Can you work these out from the model? Positions are in its coordinate system, mm. Round coordinates to 2 decimals unless told otherwise and drop trailing zeros. One line per question, with ' | ' between items.
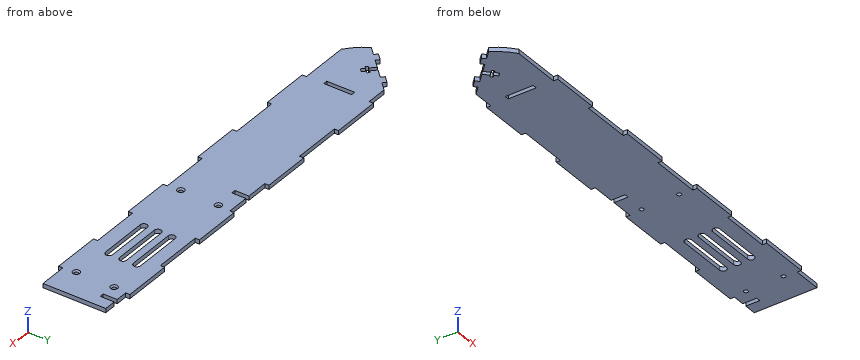
Autodesk Inventor part; units mm, degrees
ref_plane "YZ Plane" through (0, 0, 0) normal (1, 0, 0) x (0, 1, 0)
ref_plane "XZ Plane" through (0, 0, 0) normal (0, 1, 0) x (-1, 0, 0)
ref_plane "XY Plane" through (0, 0, 0) normal (0, 0, 1) x (1, 0, 0)
sketch "Sketch1" plane through (0, 0, 0) normal (0, 0, 1) x (1, 0, 0)
  line L0 (142.5, -22.5) -> (142.5, 22.5)
  arc A0 (-169.3198, -9.3198) -> (-157.5, -22.5) centre (-130.5627, 13.547) ccw
  line L1 (-154.4706, 5.5294) -> (-150.935, 1.9939)
  line L2 (-150.935, 1.9939) -> (-152.2157, 0.7132)
  line L3 (-152.2157, 0.7132) -> (-150.8015, -0.701)
  line L4 (-150.8015, -0.701) -> (-149.5208, 0.5797)
  line L5 (-149.5208, 0.5797) -> (-147.3995, -1.5416)
  line L6 (-147.3995, -1.5416) -> (-145.2782, 0.5797)
  line L7 (-145.2782, 0.5797) -> (-147.3995, 2.701)
  line L8 (-147.3995, 2.701) -> (-146.1188, 3.9817)
  line L9 (-146.1188, 3.9817) -> (-147.533, 5.3959)
  line L10 (-147.533, 5.3959) -> (-148.8137, 4.1152)
  line L11 (-148.8137, 4.1152) -> (-152.3492, 7.6508)
  line L12 (-154.542, 7.7222) -> (-156.666, 9.8462) construction
  line L13 (-122.5, 22.5) -> (-122.5, 25.5)
  line L14 (-122.5, 25.5) -> (-87.5, 25.5)
  line L15 (-87.5, 25.5) -> (-87.5, 22.5)
  line L16 (-52.5, 22.5) -> (-52.5, 25.5)
  line L17 (-52.5, 25.5) -> (-17.5, 25.5)
  line L18 (-17.5, 25.5) -> (-17.5, 22.5)
  line L19 (17.5, 22.5) -> (17.5, 25.5)
  line L20 (17.5, 25.5) -> (52.5, 25.5)
  line L21 (52.5, 25.5) -> (52.5, 22.5)
  line L22 (87.5, 22.5) -> (87.5, 25.5)
  line L23 (87.5, 25.5) -> (122.5, 25.5)
  line L24 (122.5, 25.5) -> (122.5, 22.5)
  line L25 (87.5, 22.5) -> (52.5, 22.5)
  line L26 (-52.5, 22.5) -> (-87.5, 22.5)
  line L27 (-122.5, 22.5) -> (-137.5, 22.5)
  line L28 (-122.5, -22.5) -> (-122.5, -25.5)
  line L29 (-122.5, -25.5) -> (-87.5, -25.5)
  line L30 (-87.5, -25.5) -> (-87.5, -22.5)
  line L31 (-52.5, -22.5) -> (-52.5, -25.5)
  line L32 (-52.5, -25.5) -> (-17.5, -25.5)
  line L33 (-17.5, -25.5) -> (-17.5, -22.5)
  line L34 (17.5, -22.5) -> (17.5, -25.5)
  line L35 (17.5, -25.5) -> (52.5, -25.5)
  line L36 (52.5, -25.5) -> (52.5, -22.5)
  line L37 (87.5, -22.5) -> (87.5, -25.5)
  line L38 (87.5, -25.5) -> (122.5, -25.5)
  line L39 (122.5, -25.5) -> (122.5, -22.5)
  line L40 (-157.5, -22.5) -> (-122.5, -22.5)
  line L41 (-87.5, -22.5) -> (-52.5, -22.5)
  line L42 (-17.5, -22.5) -> (17.5, -22.5)
  line L43 (52.5, -22.5) -> (87.5, -22.5)
  line L44 (122.5, -22.5) -> (142.5, -22.5)
  line L45 (-1.5, 12.5) -> (-1.5, 22.5)
  line L46 (1.5, 22.5) -> (1.5, 12.5)
  line L47 (1.5, 12.5) -> (-1.5, 12.5)
  line L48 (-37.337, 0) -> (-30.889, 0) construction
  line L49 (-164.0165, -4.0165) -> (-166.1378, -1.8952)
  line L50 (-166.1378, -1.8952) -> (-161.8952, 2.3475)
  line L51 (-161.8952, 2.3475) -> (-159.7739, 0.2261)
  line L52 (-147.0459, 12.9541) -> (-149.1673, 15.0754)
  line L53 (-149.1673, 15.0754) -> (-144.9246, 19.318)
  line L54 (-144.9246, 19.318) -> (-142.8033, 17.1967)
  line L55 (-154.4706, 5.5294) -> (-159.7739, 0.2261)
  line L56 (-164.0165, -4.0165) -> (-169.3198, -9.3198)
  line L57 (-137.5, 22.5) -> (-142.8033, 17.1967)
  line L58 (-147.0459, 12.9541) -> (-152.3492, 7.6508)
  line L59 (17.5, 22.5) -> (1.5, 22.5)
  line L60 (-1.5, 22.5) -> (-17.5, 22.5)
  line L61 (131, 22.5) -> (131, 12.5)
  line L62 (131, 12.5) -> (134, 12.5)
  line L63 (134, 12.5) -> (134, 22.5)
  line L64 (122.5, 22.5) -> (131, 22.5)
  line L65 (134, 22.5) -> (142.5, 22.5)
  point P0 (0, 0)
  point P1 (142.5, 0)
  point P2 (-146.3388, -0.481)
  point P3 (0, -22.5)
  point P4 (1.5, -22.5)
  dimension "d0" = 45
  dimension "d2" = 45
  dimension "d4" = 45
  dimension "d7" = 3
  dimension "d8" = 2
  dimension "d9" = 3
  dimension "d10" = 5
  dimension "d11" = 6.6223
  dimension "d13" = 35
  dimension "d15" = 20
  dimension "d17" = 10
  dimension "d23" = 45
  dimension "d24" = 6
  dimension "d25" = 18
  dimension "d35" = 3
  dimension "d36" = 35
  dimension "d37" = 15
  dimension "d38" = 300
  dimension "d40" = 8.5
extrude "Extrusion1" add sketch "Sketch1" along normal blind 3
sketch "Sketch2" plane through (0, 0, 3) normal (0, 0, 1) x (1, 0, 0)
  line L0 (1.5, 22.5) -> (1.5, 12.5)
  line L1 (142.5, -22.5) -> (142.5, 22.5)
  line L2 (122.5, 22.5) -> (122.5, 25.5)
  line L3 (122.5, 25.5) -> (87.5, 25.5)
  line L4 (87.5, 25.5) -> (87.5, 22.5)
  line L5 (87.5, 22.5) -> (52.5, 22.5)
  line L6 (52.5, 22.5) -> (52.5, 25.5)
  line L7 (52.5, 25.5) -> (17.5, 25.5)
  line L8 (17.5, 25.5) -> (17.5, 22.5)
  line L9 (17.5, 22.5) -> (1.5, 22.5)
  line L10 (-17.5, -22.5) -> (17.5, -22.5)
  line L11 (17.5, -22.5) -> (17.5, -25.5)
  line L12 (17.5, -25.5) -> (52.5, -25.5)
  line L13 (52.5, -25.5) -> (52.5, -22.5)
  line L14 (52.5, -22.5) -> (87.5, -22.5)
  line L15 (87.5, -22.5) -> (87.5, -25.5)
  line L16 (87.5, -25.5) -> (122.5, -25.5)
  line L17 (122.5, -25.5) -> (122.5, -22.5)
  line L18 (122.5, -22.5) -> (142.5, -22.5)
  line L19 (-125.5, 10) -> (-125.5, -10)
  line L20 (131, 22.5) -> (122.5, 22.5)
  line L21 (1.5, 12.5) -> (-1.5, 12.5)
  line L22 (-1.5, 12.5) -> (-1.5, 22.5)
  line L23 (-1.5, 22.5) -> (-17.5, 22.5)
  line L24 (-17.5, 22.5) -> (-17.5, 25.5)
  line L25 (-17.5, 25.5) -> (-52.5, 25.5)
  line L26 (-52.5, 25.5) -> (-52.5, 22.5)
  line L27 (-52.5, 22.5) -> (-87.5, 22.5)
  line L28 (-87.5, 22.5) -> (-87.5, 25.5)
  line L29 (-87.5, 25.5) -> (-122.5, 25.5)
  line L30 (-122.5, 25.5) -> (-122.5, 22.5)
  line L31 (-122.5, -25.5) -> (-87.5, -25.5)
  line L32 (-87.5, -25.5) -> (-87.5, -22.5)
  line L33 (-87.5, -22.5) -> (-52.5, -22.5)
  line L34 (-52.5, -22.5) -> (-52.5, -25.5)
  line L35 (-52.5, -25.5) -> (-17.5, -25.5)
  line L36 (-17.5, -25.5) -> (-17.5, -22.5)
  line L37 (-122.5, 22.5) -> (-137.5, 22.5)
  line L38 (-137.5, 22.5) -> (-142.8033, 17.1967)
  line L39 (-142.8033, 17.1967) -> (-144.9246, 19.318)
  line L40 (-144.9246, 19.318) -> (-149.1673, 15.0754)
  line L41 (-149.1673, 15.0754) -> (-147.0459, 12.9541)
  line L42 (-147.0459, 12.9541) -> (-152.3492, 7.6508)
  line L43 (-152.3492, 7.6508) -> (-148.8137, 4.1152)
  line L44 (-148.8137, 4.1152) -> (-147.533, 5.3959)
  line L45 (-147.533, 5.3959) -> (-146.1188, 3.9817)
  line L46 (-146.1188, 3.9817) -> (-147.3995, 2.701)
  line L47 (-147.3995, 2.701) -> (-145.2782, 0.5797)
  line L48 (-157.5, -22.5) -> (-122.5, -22.5)
  line L49 (-122.5, -22.5) -> (-122.5, -25.5)
  line L50 (-145.2782, 0.5797) -> (-147.3995, -1.5416)
  line L51 (-147.3995, -1.5416) -> (-149.5208, 0.5797)
  line L52 (-149.5208, 0.5797) -> (-150.8015, -0.701)
  line L53 (-150.8015, -0.701) -> (-152.2157, 0.7132)
  line L54 (-152.2157, 0.7132) -> (-150.935, 1.9939)
  line L55 (-150.935, 1.9939) -> (-154.4706, 5.5294)
  line L56 (-154.4706, 5.5294) -> (-159.7739, 0.2261)
  line L57 (-159.7739, 0.2261) -> (-161.8952, 2.3475)
  line L58 (-161.8952, 2.3475) -> (-166.1378, -1.8952)
  line L59 (-166.1378, -1.8952) -> (-164.0165, -4.0165)
  line L60 (-164.0165, -4.0165) -> (-169.3198, -9.3198)
  arc A0 (-169.3198, -9.3198) -> (-157.5, -22.5) centre (-130.5627, 13.547) ccw
  line L61 (142.5, 22.5) -> (134, 22.5)
  line L62 (134, 22.5) -> (134, 12.5)
  line L63 (134, 12.5) -> (131, 12.5)
  line L64 (131, 12.5) -> (131, 22.5)
  line L65 (-125.5, 10) -> (-122.5, 10)
  line L66 (-122.5, 10) -> (-122.5, -10)
  line L67 (-122.5, -10) -> (-125.5, -10)
  line L68 (-87.5, 22.5) -> (-87.5, 25.5)
  point P0 (0, 0)
  point P1 (-125.5, 0)
  dimension "d20" = 268
  dimension "d39" = 20
extrude "Extrusion2" cut sketch "Sketch2" against normal blind 10 contours L65 L66 L67 L19
sketch "Sketch3" plane through (0, 0, 3) normal (0, 0, 1) x (1, 0, 0)
  line L0 (1.5, 22.5) -> (1.5, 12.5)
  line L1 (142.5, -22.5) -> (142.5, 22.5)
  line L2 (122.5, 22.5) -> (122.5, 25.5)
  line L3 (122.5, 25.5) -> (87.5, 25.5)
  line L4 (87.5, 25.5) -> (87.5, 22.5)
  line L5 (87.5, 22.5) -> (52.5, 22.5)
  line L6 (52.5, 22.5) -> (52.5, 25.5)
  line L7 (52.5, 25.5) -> (17.5, 25.5)
  line L8 (17.5, 25.5) -> (17.5, 22.5)
  line L9 (17.5, 22.5) -> (1.5, 22.5)
  line L10 (-17.5, -22.5) -> (17.5, -22.5)
  line L11 (17.5, -22.5) -> (17.5, -25.5)
  line L12 (17.5, -25.5) -> (52.5, -25.5)
  line L13 (52.5, -25.5) -> (52.5, -22.5)
  line L14 (52.5, -22.5) -> (87.5, -22.5)
  line L15 (87.5, -22.5) -> (87.5, -25.5)
  line L16 (87.5, -25.5) -> (122.5, -25.5)
  line L17 (122.5, -25.5) -> (122.5, -22.5)
  line L18 (122.5, -22.5) -> (142.5, -22.5)
  arc A0 (59.5166, -6.8198) -> (59.5166, -11.8198) centre (59.5166, -9.3198) ccw
  arc A1 (94.5166, -11.8198) -> (94.5166, -6.8198) centre (94.5166, -9.3198) ccw
  line L19 (59.5166, -6.8198) -> (94.5166, -6.8198)
  line L20 (59.5166, -11.8198) -> (94.5166, -11.8198)
  line L21 (131, 22.5) -> (122.5, 22.5)
  line L22 (1.5, 12.5) -> (-1.5, 12.5)
  line L23 (-1.5, 12.5) -> (-1.5, 22.5)
  line L24 (-1.5, 22.5) -> (-17.5, 22.5)
  line L25 (-17.5, 22.5) -> (-17.5, 25.5)
  line L26 (-17.5, 25.5) -> (-52.5, 25.5)
  line L27 (-52.5, 25.5) -> (-52.5, 22.5)
  line L28 (-52.5, 22.5) -> (-87.5, 22.5)
  line L29 (-87.5, 22.5) -> (-87.5, 25.5)
  line L30 (-87.5, 25.5) -> (-122.5, 25.5)
  line L31 (-122.5, -22.5) -> (-122.5, -25.5)
  line L32 (-122.5, -25.5) -> (-87.5, -25.5)
  line L33 (-87.5, -25.5) -> (-87.5, -22.5)
  line L34 (-87.5, -22.5) -> (-52.5, -22.5)
  line L35 (-52.5, -22.5) -> (-52.5, -25.5)
  line L36 (-52.5, -25.5) -> (-17.5, -25.5)
  line L37 (-17.5, -25.5) -> (-17.5, -22.5)
  line L38 (-122.5, 22.5) -> (-137.5, 22.5)
  line L39 (-137.5, 22.5) -> (-142.8033, 17.1967)
  line L40 (-142.8033, 17.1967) -> (-144.9246, 19.318)
  line L41 (-144.9246, 19.318) -> (-149.1673, 15.0754)
  line L42 (-149.1673, 15.0754) -> (-147.0459, 12.9541)
  line L43 (-147.0459, 12.9541) -> (-152.3492, 7.6508)
  line L44 (-157.5, -22.5) -> (-122.5, -22.5)
  line L45 (-164.0165, -4.0165) -> (-169.3198, -9.3198)
  arc A2 (-169.3198, -9.3198) -> (-157.5, -22.5) centre (-130.5627, 13.547) ccw
  line L46 (-125.5, -10) -> (-125.5, 10)
  line L47 (142.5, 22.5) -> (134, 22.5)
  line L48 (134, 22.5) -> (134, 12.5)
  line L49 (134, 12.5) -> (131, 12.5)
  line L50 (131, 12.5) -> (131, 22.5)
  line L51 (-122.5, -10) -> (-125.5, -10)
  line L52 (-125.5, 10) -> (-122.5, 10)
  line L53 (-122.5, 10) -> (-122.5, -10)
  line L54 (-152.3492, 7.6508) -> (-148.8137, 4.1152)
  line L55 (-148.8137, 4.1152) -> (-147.533, 5.3959)
  line L56 (-147.533, 5.3959) -> (-146.1188, 3.9817)
  line L57 (-146.1188, 3.9817) -> (-147.3995, 2.701)
  line L58 (-147.3995, 2.701) -> (-145.2782, 0.5797)
  line L59 (-145.2782, 0.5797) -> (-147.3995, -1.5416)
  line L60 (-147.3995, -1.5416) -> (-149.5208, 0.5797)
  line L61 (-149.5208, 0.5797) -> (-150.8015, -0.701)
  line L62 (-150.8015, -0.701) -> (-152.2157, 0.7132)
  line L63 (-152.2157, 0.7132) -> (-150.935, 1.9939)
  line L64 (-150.935, 1.9939) -> (-154.4706, 5.5294)
  line L65 (-154.4706, 5.5294) -> (-159.7739, 0.2261)
  line L66 (-159.7739, 0.2261) -> (-161.8952, 2.3475)
  line L67 (-161.8952, 2.3475) -> (-166.1378, -1.8952)
  line L68 (-166.1378, -1.8952) -> (-164.0165, -4.0165)
  line L69 (-122.5, 25.5) -> (-122.5, 22.5)
  point P0 (0, 0)
  dimension "d26" = 5
  dimension "d27" = 35
extrude "Extrusion3" cut sketch "Sketch3" against normal up to next contours L19 A1 L20 A0
pattern_linear "Rectangular Pattern1" count 3 spacing 10 along (0, 1, 0) of "Extrusion3"
sketch "Sketch4" plane through (0, 0, 3) normal (0, 0, 1) x (1, 0, 0)
  line L0 (1.5, 22.5) -> (1.5, 12.5)
  line L1 (-17.4416, 0) -> (12.3581, 0) construction
  point P0 (0, 0)
  point P1 (16.5, 13.5)
  point P2 (16.5, -13.5)
  point P3 (121.5, 13.5)
  point P4 (121.5, -13.5)
  dimension "d41" = 27
  dimension "d42" = 15
  dimension "d43" = 105
hole "Hole1" at (16.5, 13.5, 3) at (16.5, -13.5, 3) at (121.5, 13.5, 3) at (121.5, -13.5, 3) direction (0, 0, -1) diameter 3 end through all countersink diameter 5 countersink angle 90
properties part number "Wall" material "Polycarbonate, Clear"
(1) Please list where these lines run through material, in increasing order: probe 1 along X at (y, z) = (13.5, 0.6); probe 2 along Y at (x, z) = (16.5, 1.15); probe 3 along Y at (x, z) = (121.5, 0.75). Write a range as [from, to].
Final values:
probe 1: [-147.59, -1.5], [1.5, 15], [18, 120], [123, 131], [134, 142.5] | probe 2: [-22.5, -15], [-12, 12], [15, 22.5] | probe 3: [-25.5, -15], [-12, 12], [15, 25.5]
(2) Will these pins go through, and if not, where does the flat tip stop? pin 1 Ø0.9 at (x, z) = (10.5, 2) entering from +Y; pin 2 Ø1.5 at (y, z) = (-24, 1) entering from +X; pin 3 Ø1.5 at (x, z) = (71, 1) entering from -Y.
Final values:
pin 1: y = 22.5 | pin 2: x = 122.5 | pin 3: y = -22.5
(3) If we section it at A-A on z = 1.5: State how many separate pieces and enclosed holes the cut face has, plus the area to 3 significant figures.
Final values:
separate pieces: 1 | enclosed holes: 8 | area: 13,600 mm^2
